The listing builds one solid part. Answer for the finished solid, in the listing's coordinates (mm). A direction names the side the tool comes from. Coordinates: 2 decimals unless noted, no trailing zeros. Write each loop counter-clockwise with the first axis right and the second up, starting at its lowest first coordinate (ties: lowest second). Pieces come first, ordered by that corner, then holes.
(1) The part is cut by section C-C on x = -8.5. Determine the outline of the cut face in (y, z), plus the area to 3 significant figures.
(2) For a pull along X with two mould halves and no side action, classify faces 5 (the cylindrical face through (-0.54, -2.44, 12.85)), 6 (the cylindrical face through (15.66, -14.26, -6.76)), 7 (the flat face through (21.209, 0, -3)), 8 (the flat face through (-21.109, 0, -16)) as +X half, -X half, draft (parallel to the pull), parting line (faces both ways), or undercut.
(3) Straight lines are drawn through the part: line 1 (Y direction, x = -15.5, z = -2.4); line 2 (Y direction, x = 15, z = -3); line 3 (X direction, y = 15.5, z = -6.4). For each, find the intervals that lie inside material, in ascending order.
(4) The part is cut by section B-B on y = 0. Determine the outline of the cut face in (x, z).
(5) Which of the six approach directions +Z, -Z, +X, -X, +Y, -Y give full straight-line access (tool end or side, diameter ignored) to faces 1 (the cylindrical face through (17.623, 17.732, -15.86)), 2 (the cylindrical face through (17.732, -17.623, -15.86)), 3 (the cylindrical face through (14, -15.43, -2.96)), 4 (the flat face through (0, 2, 16))?
(6) The part is cut by section A-A on z = -11. Determine the outline of the cut face in (x, y), plus the area to 3 significant figures.
(7) The part is cut by section D-D on y = -9. Determine the outline of the cut face in (x, z), plus the area to 3 significant figures.
(8) Given P1, Ø6, axis at x = 5.5, z = -17.5, coming from the +Y side; P2, Ø2.5, axis at x = 15, y = -16, coming from the +Z side; P3, Ø12, axis at x = -12, z = 14, coming from the +Y side; P4, Ø12, axis at y = -2, z = -17, coming from the -X side, each flat-ended and moving along its own axis, determine where each tip first touches the part or whether it passes through.
from build123d import *

# Parameters (mm, degrees)
SKETCH1_R                       = 2.5
BOSS_EXTRUDE1_DEPTH             = 24
SKETCH2_R                       = 11
BOSS_EXTRUDE2_DEPTH             = 2
SKETCH3_W                       = 42.418
SKETCH3_H                       = 42.418
BOSS_EXTRUDE3_DEPTH             = 32
CUT_EXTRUDE1_DEPTH              = 64.526713767
M3X0_5_TAPPED_HOLE1_D           = 2.5
M3X0_5_TAPPED_HOLE1_DEPTH       = 7.5
M3X0_5_TAPPED_HOLE1_CBORE_D     = 3
M3X0_5_TAPPED_HOLE1_CBORE_DEPTH = 6
M3X0_5_TAPPED_HOLE1_TIP         = 0.751075774
CUT_EXTRUDE2_START              = -15
CUT_EXTRUDE2_DEPTH              = 15
CUT_EXTRUDE3_DEPTH              = 10


with BuildPart() as part:
    # Sketch1 → Boss-Extrude1 (new body)
    with BuildSketch(Plane.XY):
        Circle(SKETCH1_R)
    extrude(amount=BOSS_EXTRUDE1_DEPTH)

    # Sketch2 → Boss-Extrude2 (add)
    with BuildSketch(Plane(origin=(0, 0, 0), x_dir=(-1, 0, 0), z_dir=(0, 0, -1))):
        Circle(SKETCH2_R)
    extrude(amount=-BOSS_EXTRUDE2_DEPTH)

    # Sketch3 → Boss-Extrude3 (add)
    with BuildSketch(Plane(origin=(0, 0, 0), x_dir=(-1, 0, 0), z_dir=(0, 0, -1))):
        Rectangle(SKETCH3_W, SKETCH3_H)
    extrude(amount=BOSS_EXTRUDE3_DEPTH)

    # Sketch4 → Cut-Extrude1 (cut, through all)
    with BuildSketch(Plane(origin=(0, 0, -32), x_dir=(-1, 0, 0), z_dir=(0, 0, -1))):
        with BuildLine():
            Line((-21.209, -15.887992919), (-21.209, -21.209))
            Line((-21.209, -21.209), (-15.887992919, -21.209))
            ThreePointArc((-15.887992919, -21.209), (-18.738329701, -18.738329701), (-21.209, -15.887992919))
        make_face()
        with BuildLine():
            Line((15.887992919, -21.209), (21.209, -21.209))
            Line((21.209, -21.209), (21.209, -15.887992919))
            ThreePointArc((21.209, -15.887992919), (18.738329701, -18.738329701), (15.887992919, -21.209))
        make_face()
        with BuildLine():
            Line((21.209, 15.887992919), (21.209, 21.209))
            Line((21.209, 21.209), (15.887992919, 21.209))
            ThreePointArc((15.887992919, 21.209), (18.738329701, 18.738329701), (21.209, 15.887992919))
        make_face()
        with BuildLine():
            Line((-15.887992919, 21.209), (-21.209, 21.209))
            Line((-21.209, 21.209), (-21.209, 15.887992919))
            ThreePointArc((-21.209, 15.887992919), (-18.738329701, 18.738329701), (-15.887992919, 21.209))
        make_face()
    extrude(amount=-CUT_EXTRUDE1_DEPTH, mode=Mode.SUBTRACT)

    # M3x0.5 Tapped Hole1
    with Locations(Plane.XY):
        with Locations((-15.5, 15.5), (-15.5, -15.5), (15.5, -15.5), (15.5, 15.5)):
            CounterBoreHole(M3X0_5_TAPPED_HOLE1_D / 2, M3X0_5_TAPPED_HOLE1_CBORE_D / 2, M3X0_5_TAPPED_HOLE1_CBORE_DEPTH, depth=M3X0_5_TAPPED_HOLE1_DEPTH)
            with Locations((0, 0, -(M3X0_5_TAPPED_HOLE1_DEPTH + M3X0_5_TAPPED_HOLE1_TIP / 2))):  # 118° drill point
                Cone(0, M3X0_5_TAPPED_HOLE1_D / 2, M3X0_5_TAPPED_HOLE1_TIP, mode=Mode.SUBTRACT)

    # Sketch7 → Cut-Extrude2 (cut)
    with BuildSketch(Plane.XY.offset(24).offset(CUT_EXTRUDE2_START)):
        with BuildLine():
            Line((-1.5, 2), (1.5, 2))
            ThreePointArc((1.5, 2), (0, 2.5), (-1.5, 2))
        make_face()
    extrude(amount=CUT_EXTRUDE2_DEPTH, mode=Mode.SUBTRACT)

    # Sketch8 → Cut-Extrude3 (cut, symmetric)
    with BuildSketch(Plane.XY.offset(-16)):
        with BuildLine():
            Line((15.887992919, 21.209), (-15.887992919, 21.209))
            ThreePointArc((-15.887992919, 21.209), (-18.738329701, 18.738329701), (-21.209, 15.887992919))
            Line((-21.209, 15.887992919), (-21.209, -15.887992919))
            ThreePointArc((-21.209, -15.887992919), (-18.738329701, -18.738329701), (-15.887992919, -21.209))
            Line((-15.887992919, -21.209), (15.887992919, -21.209))
            ThreePointArc((15.887992919, -21.209), (18.738329701, -18.738329701), (21.209, -15.887992919))
            Line((21.209, -15.887992919), (21.209, 15.887992919))
            ThreePointArc((21.209, 15.887992919), (18.738329701, 18.738329701), (15.887992919, 21.209))
        make_face()
        with BuildLine():
            Line((-13.394406258, 21.109), (13.394406258, 21.109))
            ThreePointArc((13.394406258, 21.109), (17.67766953, 17.67766953), (21.109, 13.394406258))
            Line((21.109, 13.394406258), (21.109, -13.394406258))
            ThreePointArc((21.109, -13.394406258), (17.67766953, -17.67766953), (13.394406258, -21.109))
            Line((13.394406258, -21.109), (-13.394406258, -21.109))
            ThreePointArc((-13.394406258, -21.109), (-17.67766953, -17.67766953), (-21.109, -13.394406258))
            Line((-21.109, -13.394406258), (-21.109, 13.394406258))
            ThreePointArc((-21.109, 13.394406258), (-17.67766953, 17.67766953), (-13.394406258, 21.109))
        make_face(mode=Mode.SUBTRACT)
    extrude(amount=CUT_EXTRUDE3_DEPTH, both=True, mode=Mode.SUBTRACT)


solid = part.part
Model answer:
1. outline: (-21.21, -32) - (21.21, -32) - (21.21, -26) - (21.11, -26) - (21.11, -6) - (21.21, -6) - (21.21, 0) - (6.98, 0) - (6.98, 2) - (-6.98, 2) - (-6.98, 0) - (-21.21, 0) - (-21.21, -6) - (-21.11, -6) - (-21.11, -26) - (-21.21, -26) - close
1. area: 1,380 mm2
2. face 5: parting line
2. face 6: undercut
2. face 7: +X half
2. face 8: -X half
3. line 1: y = -21.21 to -17, -14 to 14, 17 to 21.21
3. line 2: y = -21.21 to -16.91, -14.09 to 14.09, 16.91 to 21.21
3. line 3: x = -19.62 to -16.75, -14.25 to 14.25, 16.75 to 19.62
4. outline: (-21.21, -32) - (21.21, -32) - (21.21, -26) - (21.11, -26) - (21.11, -6) - (21.21, -6) - (21.21, 0) - (11, 0) - (11, 2) - (2.5, 2) - (2.5, 24) - (-2.5, 24) - (-2.5, 2) - (-11, 2) - (-11, 0) - (-21.21, 0) - (-21.21, -6) - (-21.11, -6) - (-21.11, -26) - (-21.21, -26) - close
5. face 1: +X, +Y
5. face 2: +X, -Y
5. face 3: +Z
5. face 4: +Z, +X, -X, +Y
6. outline: (-21.11, -13.39) arc R25 ccw to (-13.39, -21.11) - (13.39, -21.11) arc R25 ccw to (21.11, -13.39) - (21.11, 13.39) arc R25 ccw to (13.39, 21.11) - (-13.39, 21.11) arc R25 ccw to (-21.11, 13.39) - close
6. area: 1,680 mm2
7. outline: (-21.21, -32) - (21.21, -32) - (21.21, -26) - (21.11, -26) - (21.11, -6) - (21.21, -6) - (21.21, 0) - (6.32, 0) - (6.32, 2) - (-6.32, 2) - (-6.32, 0) - (-21.21, 0) - (-21.21, -6) - (-21.11, -6) - (-21.11, -26) - (-21.21, -26) - close
7. area: 1,380 mm2
8. P1: stops at y = 21.11
8. P2: stops at z = 0
8. P3: passes through
8. P4: stops at x = -21.11
